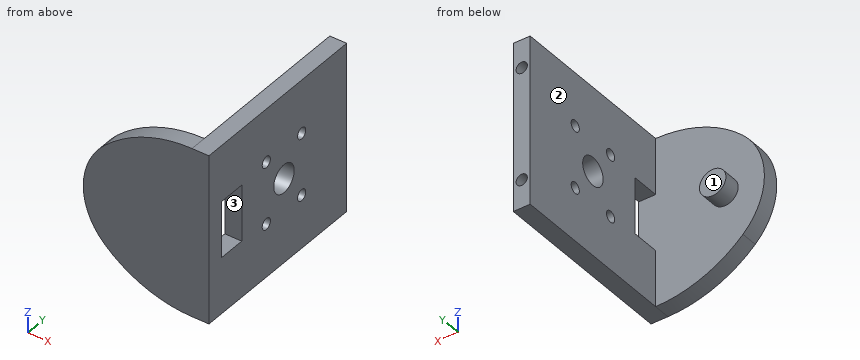
```python
from build123d import *

# Parameters (mm, degrees)
BOSS_EXTRUDE1_DEPTH     = 3
ESQUISSE1_W             = 3
ESQUISSE1_H             = 30
BOSS_EXTRU_1_DEPTH      = 30.6
ESQUISSE2_R             = 1
ENL_V_MAT_EXTRU_1_DEPTH = 3
ESQUISSE3_R             = 2.35
BOSS_EXTRU_2_DEPTH      = 3
ESQUISSE4_R             = 2.5
ENL_V_MAT_EXTRU_2_DEPTH = 40.164397097
ESQUISSE5_R             = 1
ENL_V_MAT_EXTRU_3_DEPTH = 10
SKETCH2_W               = 10
SKETCH2_H               = 5
CUT_EXTRUDE1_DEPTH      = 40.164397097


with BuildPart() as part:
    # Sketch1 → Boss-Extrude1 (new body)
    with BuildSketch(Plane(origin=(0, 0, 0), x_dir=(1, 0, 0), z_dir=(0, 1, 0))):
        with BuildLine():
            Line((15.3, 15), (12.3, 15))
            ThreePointArc((12.3, 15), (3.958234572, 13.40032808), (-3.2, 8.828273999))
            ThreePointArc((-3.2, 8.828273999), (-7, 0), (-3.2, -8.828273999))
            ThreePointArc((-3.2, -8.828273999), (3.958234572, -13.40032808), (12.3, -15))
            Line((12.3, -15), (15.3, -15))
            Line((15.3, -15), (15.3, 15))
        make_face()
    extrude(amount=-BOSS_EXTRUDE1_DEPTH)

    # Esquisse1 → Boss.-Extru.1 (add)
    with BuildSketch(Plane(origin=(0, 0, 0), x_dir=(1, 0, 0), z_dir=(0, 1, 0))):
        with Locations((13.8, 0)):
            Rectangle(ESQUISSE1_W, ESQUISSE1_H)
    extrude(amount=BOSS_EXTRU_1_DEPTH)

    # Esquisse2 → Enlèv. mat.-Extru.1 (cut)
    with BuildSketch(Plane(origin=(0, 30.6, 0), x_dir=(1, 0, 0), z_dir=(0, 1, 0))):
        with Locations(Location((13.8, 10, 0), (0, 0, 270))):
            Circle(ESQUISSE2_R)
        with Locations(Location((13.8, -10, 0), (0, 0, 270))):
            Circle(ESQUISSE2_R)
    extrude(amount=-ENL_V_MAT_EXTRU_1_DEPTH, mode=Mode.SUBTRACT)

    # Esquisse3 → Boss.-Extru.2 (add)
    with BuildSketch(Plane(origin=(0, 0, 0), x_dir=(1, 0, 0), z_dir=(0, 1, 0))):
        with Locations(Location((0, 0, 0), (0, 0, 270))):
            Circle(ESQUISSE3_R)
    extrude(amount=BOSS_EXTRU_2_DEPTH)

    # Esquisse4 → Enlèv. mat.-Extru.2 (cut, through all)
    with BuildSketch(Plane.ZY.offset(-12.3)):
        with Locations((0, 15.3)):
            Circle(ESQUISSE4_R)
    extrude(amount=-ENL_V_MAT_EXTRU_2_DEPTH, mode=Mode.SUBTRACT)

    # Esquisse5 → Enlèv. mat.-Extru.3 (cut)
    with BuildSketch(Plane(origin=(15.3, 0, 0), x_dir=(0, 0, -1), z_dir=(1, 0, 0))):
        with Locations((5.516503864, 19.609081703)):
            Circle(ESQUISSE5_R)
        with Locations((5.515646632, 10.989821091)):
            Circle(ESQUISSE5_R)
        with Locations((-5.515646632, 19.610178909)):
            Circle(ESQUISSE5_R)
        with Locations((-5.516503864, 10.990918297)):
            Circle(ESQUISSE5_R)
    extrude(amount=-ENL_V_MAT_EXTRU_3_DEPTH, mode=Mode.SUBTRACT)

    # Sketch2 → Cut-Extrude1 (cut, through all)
    with BuildSketch(Plane.ZY.offset(-12.3)):
        with Locations((0, 2.5)):
            Rectangle(SKETCH2_W, SKETCH2_H)
    extrude(amount=-CUT_EXTRUDE1_DEPTH, mode=Mode.SUBTRACT)


solid = part.part
```
Build history of the part. All positions in model axes, mm. Face numbers are marked on the shaded views. Give positions to 0.01 mm unless a question says otherwise; leave off trailing zeros. Order: outer loops, then holes, each group sorted by start corner. A loop starts at its lowest first (then second) coordinate and runs counter-clockwise, first axis right, second up. Notation, with made-up numbers: M 52.25,-26 L 78.25,-26 A18 cw 78.25,-7 Z; hole C 33.25,9 d11. An arc over 180 degrees is marked long. Return JSON: item names as keys, results as strings.
Q1. Flat gauge pins, fed straight in: pin 1 (1.6 mm diameter, centred on x = 13.8, z = 10, fed in from +Y); pin 2 (3 mm diameter, centred on y = 15.3, z = 0, fed in from +X); pin 3 (5 mm diameter, centred on x = -0.5, z = 0.5, fed in from +Y); pin 4 (2 mm diameter, centred on x = 3.5, z = -9.5, fed in from +Y). Where does each tip first touch, or does it go through?
Answer list:
{"pin 1": "stops at y = 27.6", "pin 2": "passes through", "pin 3": "stops at y = 3", "pin 4": "stops at y = 0"}
Q2. Band-saw the part on C-C (x = 0). Give the cut face in (y, z).
Answer list:
{"outline": "M -3,-11.35 L 0,-11.35 L 0,-2.35 L 3,-2.35 L 3,2.35 L 0,2.35 L 0,11.35 L -3,11.35 Z"}
Q3. Band-saw the part on D-D (x = 13.8). Give the cut face in (y, z).
Answer list:
{"outline": "M -3,-15 L 30.6,-15 L 30.6,-11 L 27.6,-11 L 27.6,-9 L 30.6,-9 L 30.6,9 L 27.6,9 L 27.6,11 L 30.6,11 L 30.6,15 L -3,15 Z; hole M 0,-5 L 5,-5 L 5,5 L 0,5 Z; hole C 10.99,-5.52 d2; hole C 10.99,5.52 d2; hole C 15.3,0 d5; hole C 19.61,-5.52 d2; hole C 19.61,5.52 d2"}
Q4. Two-plate mould, pull along Y, no slides. Class the marked faces 1, 2 and 3: pulls with the +Y half, pulls with the -Y half, needs draft (parallel to the pull), parting line crosses it, or undercut.
Answer list:
{"face 1": "pulls with the +Y half", "face 2": "needs draft", "face 3": "undercut"}
Q5. Band-saw the part on B-B (z = 0). Give the cut face in (x, y).
Answer list:
{"outline": "M -7,-3 L 15.3,-3 L 15.3,0 L 2.35,0 L 2.35,3 L -2.35,3 L -2.35,0 L -7,0 Z; M 12.3,5 L 15.3,5 L 15.3,12.8 L 12.3,12.8 Z; M 12.3,17.8 L 15.3,17.8 L 15.3,30.6 L 12.3,30.6 Z"}
Q6. Band-saw the part on A-A (y = 15.3). Give the cut face in (x, z).
Answer list:
{"outline": "M 12.3,-15 L 15.3,-15 L 15.3,-2.5 L 12.3,-2.5 Z; M 12.3,2.5 L 15.3,2.5 L 15.3,15 L 12.3,15 Z"}
Q7. Wall check: probe 1 along X at (y, z) = (28.3, -10); probe 2 along Y at (x, z) = (14.25, -3.25); probe 3 along Z at (x, y) = (14, 10.5). Give the ranges that are in metal, low to high. Write a range as from..to.
Answer list:
{"probe 1": "x = 12.3..12.8, 14.8..15.3", "probe 2": "y = -3..0, 5..30.6", "probe 3": "z = -15..-6.39, -4.64..4.65, 6.39..15"}
